```python
from build123d import *

# Parameters (mm, degrees)
CROQUIS1_R                   = 30
SALIENTE_EXTRUIR1_DEPTH      = 30
CROQUIS1_W                   = 20
CROQUIS1_H                   = 25
SALIENTE_EXTRUIR1_2_DEPTH    = 30
CROQUIS2_R                   = 35
CROQUIS2_R_2                 = 30
SALIENTE_EXTRUIR2_DEPTH      = 5
SALIENTE_EXTRUIR3_REACH      = 94.331
SALIENTE_EXTRUIR3_END_RADIUS = 30
CROQUIS3_R                   = 5
CROQUIS4_R                   = 10
SALIENTE_EXTRUIR4_DEPTH      = 10
CROQUIS5_R                   = 6
SALIENTE_EXTRUIR5_DEPTH      = 20
SALIENTE_EXTRUIR6_START      = 50
CROQUIS6_R                   = 10
SALIENTE_EXTRUIR6_DEPTH      = 50


with BuildPart() as part:
    # Croquis1 → Saliente-Extruir1 (new body)
    with BuildSketch(Plane.XY):
        with Locations((0, 20)):
            Circle(CROQUIS1_R)
    extrude(amount=-SALIENTE_EXTRUIR1_DEPTH)

    # Croquis2 → Saliente-Extruir2 (add)
    with BuildSketch(Plane.XY):
        with Locations((0, 20)):
            Circle(CROQUIS2_R)
        with Locations((0, 20)):
            Circle(CROQUIS2_R_2, mode=Mode.SUBTRACT)
    extrude(amount=-SALIENTE_EXTRUIR2_DEPTH)



with BuildPart() as body_2:
    # Croquis1 → Saliente-Extruir1 2 (new body)
    with BuildSketch(Plane.XY):
        with Locations((0, -37.5)):
            Rectangle(CROQUIS1_W, CROQUIS1_H)
    extrude(amount=-SALIENTE_EXTRUIR1_2_DEPTH)


with BuildPart() as part_1:
    add(part.part)

    add(body_2.part)  # Saliente-Extruir3 merges body 2
    # Saliente-Extruir3: up to this cylinder (the profile starts outside it)
    saliente_extruir3_end = Plane(origin=(0, 20, -15), z_dir=(0, 0, 1)) * Cylinder(SALIENTE_EXTRUIR3_END_RADIUS, 249.662, mode=Mode.PRIVATE)
    # Croquis3 → Saliente-Extruir3 (add, up to the surface)
    with BuildSketch(Plane(origin=(0, -25, 0), x_dir=(1, 0, 0), z_dir=(0, 1, 0)), mode=Mode.PRIVATE) as saliente_extruir3_sk1:
        with Locations(Location((0, 15, 0), (0, 0, 90))):
            Circle(CROQUIS3_R)
    saliente_extruir3_tool1 = extrude(saliente_extruir3_sk1.sketch, amount=SALIENTE_EXTRUIR3_REACH, mode=Mode.PRIVATE) - saliente_extruir3_end
    add(saliente_extruir3_tool1.solids().sort_by_distance((0, -25, -15))[0])

    # Croquis4 → Saliente-Extruir4 (add)
    with BuildSketch(Plane.XY):
        with Locations((0, -37.5)):
            Circle(CROQUIS4_R)
    extrude(amount=SALIENTE_EXTRUIR4_DEPTH)

    # Croquis5 → Saliente-Extruir5 (add)
    with BuildSketch(Plane.XY.offset(10)):
        with Locations((0, -37.5)):
            Circle(CROQUIS5_R)
    extrude(amount=SALIENTE_EXTRUIR5_DEPTH)

    # Croquis6 → Saliente-Extruir6 (add)
    with BuildSketch(Plane(origin=(0, 0, -30), x_dir=(-1, 0, 0), z_dir=(0, 0, -1)).offset(SALIENTE_EXTRUIR6_START)):
        with Locations(Location((0, -37.5, 0), (0, 0, 180))):
            Circle(CROQUIS6_R)
    extrude(amount=-SALIENTE_EXTRUIR6_DEPTH)


solid = part_1.part
```
Read the model definition and answer for the solid it produces. Units are mm, in the model's axes. A direction names the side the tool comes from. Coordinates: 2 decimals unless noted, no trailing zeros. Write each loop counter-clockwise with the first axis right and the second up, starting at its lowest first coordinate (ties: lowest second). Pieces come first, ordered by that corner, then holes. Notation, with made-up numbers: (18, 32.5) -> (30, 32.5) arc R23 ccw to (30, 66.5) -> close; hole circle Ø3 at (51, -34). An arc over 180 degrees is marked (long way). Write item = value, one per line.
(1) Given pin 1 Ø4 at (x, z) = (-27.5, -29.5) entering from +Y; pin 2 Ø1 at (x, z) = (1, -47) entering from -Y; pin 3 Ø12.5 at (y, z) = (-37.5, -15) entering from +X, each flat-ended and moving along its own axis, determine where each tip first touches the part or whether it passes through.
From the geometry:
pin_1 = 35.8
pin_2 = -47.49
pin_3 = 10
(2) For a pull along Y with two mould halves and no side action, classify faces 1 (the face through (-1.5, -17.4, -19.77)), 2 (the face through (0, -50, -15)), 3 (the face through (0, -48, -30)), 4 (the face through (-2.17, -27.74, -55.35)) as +Y half, -Y half, draft (parallel to the pull), parting line (faces both ways), or undercut.
From the geometry:
face_1 = undercut
face_2 = -Y half
face_3 = draft
face_4 = parting line
(3) Section D-D on z = -34.5 is taken. Write down the section's boundary in (x, y).
From the geometry:
outline = circle Ø20 at (0, -37.5)
(4) Which of the six approach directions +Z, -Z, +X, -X, +Y, -Y give full straight-line access (tool end or side, diameter ignored) to faces 5 (the face through (0, -48, 0)), 6 (the face through (0, -27, -30)), 7 (the face through (0, -27, 0))?
From the geometry:
face_5 = +Z, -Y
face_6 = -Z, +Y
face_7 = +Z, +Y
(5) Section A-A on z = -15 is taken. Write down the section's boundary in (x, y), plus the area to 3 significant figures.
From the geometry:
outline = (-10, -50) -> (10, -50) -> (10, -25) -> (5, -25) -> (5, -9.58) arc R30 ccw (long way) to (-5, -9.58) -> (-5, -25) -> (-10, -25) -> close
area = 3,480 mm2
(6) Section B-B on x = 0 is taken. Write down the section's boundary in (y, z), plus the area to 3 significant figures.
From the geometry:
outline = (-50, -30) -> (-47.5, -30) -> (-47.5, -80) -> (-27.5, -80) -> (-27.5, -30) -> (-25, -30) -> (-25, -20) -> (-10, -20) -> (-10, -30) -> (50, -30) -> (50, -5) -> (55, -5) -> (55, 0) -> (-15, 0) -> (-15, -5) -> (-10, -5) -> (-10, -10) -> (-25, -10) -> (-25, 0) -> (-27.5, 0) -> (-27.5, 10) -> (-31.5, 10) -> (-31.5, 30) -> (-43.5, 30) -> (-43.5, 10) -> (-47.5, 10) -> (-47.5, 0) -> (-50, 0) -> close
area = 4,190 mm2
(7) Section C-C on y = 20 is taken. Write down the section's boundary in (x, z), plus the area to 3 significant figures.
From the geometry:
outline = (-35, -5) -> (-30, -5) -> (-30, -30) -> (30, -30) -> (30, -5) -> (35, -5) -> (35, 0) -> (-35, 0) -> close
area = 1,850 mm2
(8) Straight lines are drawn through the part: L1, parallel to Z at x = 31.5, y = 26; L2, parallel to Z at x = -18, y = 20.5; L3, parallel to X at y = -29.5, z = -56.5. For each, find the intervals that lie inside material, in ascending order. Write a range as from..to.
From the geometry:
L1 = -5..0
L2 = -30..0
L3 = -6..6
